Could you check a few things on this drawing? It's one solid part, dimensions in mm from its lowest x, y, z. Give positions to 0.01 mm unless a question says otherwise; leave off trailing zeros. Loops run counter-clockwise (first coordinate to the right, second up) from the corner with the lowest first, then second, coordinate; pieces in that order, holes last. Notation, with made-up numbers: (-33, 82) -> (6, 82) arc R36 ccw to (6, 116) -> close; hole circle Ø10 at (-18, 39). An arc over 180 degrees is marked (long way). Use CSV: the item, a comma, the result in double quotes.
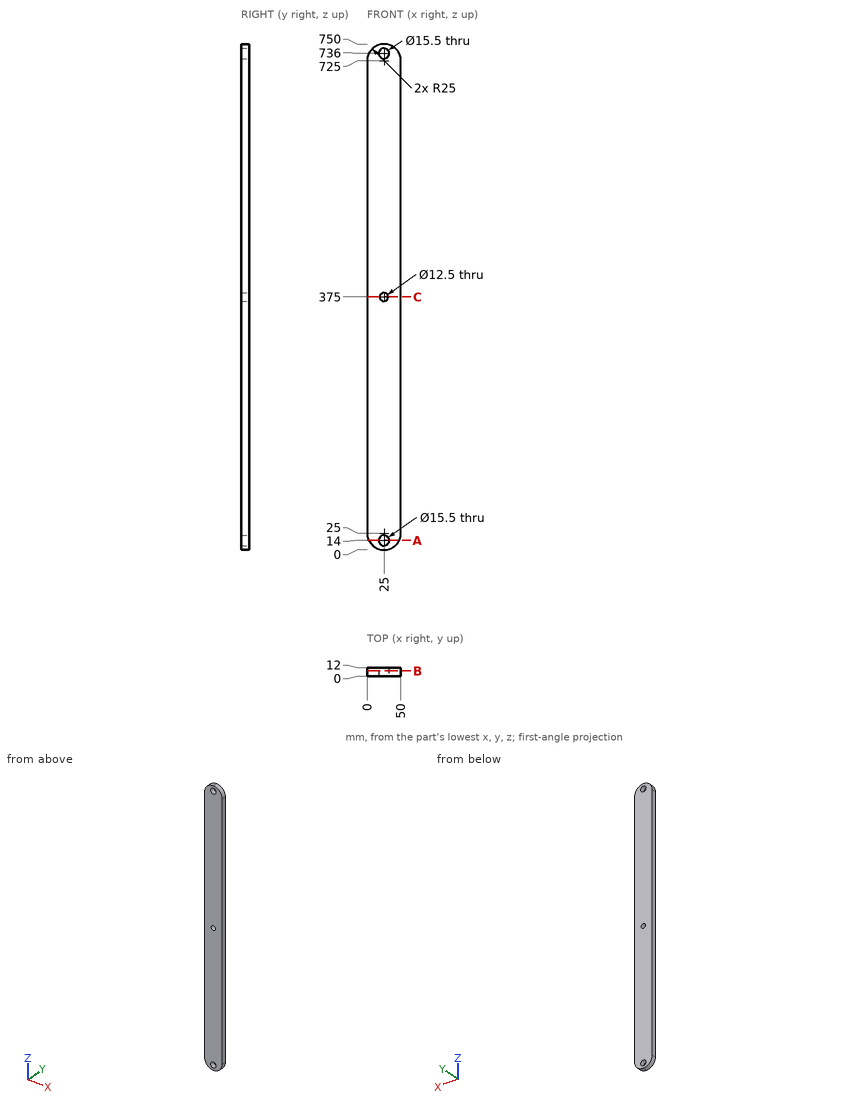
(1) If we section it at C-C, the plane z = 375: Write out the boundary of the cut face in (x, y), then the cut area to 3 significant figures.
Answer sheet:
outline,"(0, 0) -> (18.75, 0) -> (18.75, 12) -> (0, 12) -> close; (31.25, 0) -> (50, 0) -> (50, 12) -> (31.25, 12) -> close"
area,"450 mm2"
(2) If we section it at A-A, the plane z = 14: Write out the boundary of the cut face in (x, y), then the cut area to 3 significant figures.
Answer sheet:
outline,"(2.55, 0) -> (17.25, 0) -> (17.25, 12) -> (2.55, 12) -> close; (32.75, 0) -> (47.45, 0) -> (47.45, 12) -> (32.75, 12) -> close"
area,"353 mm2"
(3) If we section it at B-B, the plane y = 7.5: Write out the boundary of the cut face in (x, z).
Answer sheet:
outline,"(0, 25) arc R25 ccw to (25, 0) arc R25 ccw to (50, 25) -> (50, 725) arc R25 ccw to (25, 750) arc R25 ccw to (0, 725) -> close; hole circle Ø15.5 at (25, 14); hole circle Ø15.5 at (25, 736); hole circle Ø12.5 at (25, 375)"
(4) If I drill on L1, parallel to Z at x = 24, y = 9; L2, parallel to X at y = 7.25, z = 14; L3, parallel to X at y = 6.75, z = 375, over which ranges is the centre line in solid material (lowest first)? Write a range as from..to.
Answer sheet:
L1,"z = 0.02..6.31, 21.69..368.83, 381.17..728.31, 743.69..749.98"
L2,"x = 2.55..17.25, 32.75..47.45"
L3,"x = 0..18.75, 31.25..50"
